Autodesk Inventor part; units mm, degrees
ref_plane "YZ Plane" through (0, 0, 0) normal (1, 0, 0) x (0, 1, 0)
ref_plane "XZ Plane" through (0, 0, 0) normal (0, 1, 0) x (-1, 0, 0)
ref_plane "XY Plane" through (0, 0, 0) normal (0, 0, 1) x (1, 0, 0)
sketch "Skizze1" plane through (0, 0, 0) normal (0, 1, 0) x (-1, 0, 0)
  line L0 (18.599, 2.8535) -> (-28.901, 2.8535)
  line L1 (-28.901, 2.8535) -> (-28.901, -12.1465)
  line L2 (-28.901, -12.1465) -> (18.599, -12.1465)
  line L3 (18.599, -12.1465) -> (18.599, 2.8535)
  line L4 (18.599, -12.1465) -> (28.599, -12.1465)
  line L5 (28.599, -12.1465) -> (28.599, 2.8535)
  line L6 (28.599, 2.8535) -> (18.599, 2.8535)
  line L7 (18.599, 2.8535) -> (18.599, -12.1465)
  point P0 (0, 0)
  dimension "d0" = 47.5
  dimension "d1" = 15
  dimension "d6" = 10
extrude "Extrusion1" add sketch "Skizze1" along normal blind 10 contours L3 L2 L1 L0
sketch "Skizze2" plane through (-18.599, 0, 2.8535) normal (0, 0, 1) x (1, 0, 0)
  line L0 (47.5, 10) -> (0, 10)
  line L1 (47.5, 0) -> (0, 10)
  line L2 (0, 10) -> (47.5, 10)
  line L3 (47.5, 10) -> (47.5, 0)
  point P0 (18.599, 0)
extrude "Extrusion2" cut sketch "Skizze2" against normal up to surface (15 mm away)
sketch "Skizze3" plane through (28.901, 0, 2.8535) normal (0.206, 0.9785, 0) x (0.9785, -0.206, 0)
  point P0 (-28.2811, 2.8535)
extrude "Extrusion3" add sketch "Skizze1" along normal blind 10 contours L6 L5 L4 L3
sketch "Skizze6" plane through (-28.599, 0, 2.8535) normal (0, 0, 1) x (1, 0, 0)
  line L0 (10, 10) -> (0, 10)
  line L1 (0, 0) -> (0, 10)
  line L2 (10, 10) -> (0, 0)
  line L3 (0, 0) -> (0, 10)
  line L4 (57.5, 0) -> (10, 10)
  line L5 (0, 10) -> (10, 10)
  point P0 (28.599, 0)
extrude "Extrusion4" cut sketch "Skizze6" against normal blind 15
sketch "Skizze7" plane through (28.901, 0, 2.8535) normal (0.206, 0.9785, 0) x (0.9785, -0.206, 0)
  line L0 (0, 15) -> (-56.2666, 15)
  line L1 (-56.2666, 0) -> (0, 0)
  line L2 (-46.5412, 15) -> (-41.5412, 15)
  line L3 (-41.5412, 15) -> (-41.5412, 0)
  line L4 (-41.5412, 0) -> (-46.5412, 0)
  line L5 (-46.5412, 0) -> (-46.5412, 15)
  line L6 (-48.5412, 15) -> (-48.5412, 0)
  line L7 (-31.5412, 15) -> (-31.5412, 0)
  line L8 (-36.5412, 15) -> (-31.5412, 15)
  line L9 (-36.5412, 0) -> (-36.5412, 15)
  line L10 (-31.5412, 0) -> (-36.5412, 0)
  line L11 (-21.5412, 15) -> (-21.5412, 0)
  line L12 (-26.5412, 15) -> (-21.5412, 15)
  line L13 (-26.5412, 0) -> (-26.5412, 15)
  line L14 (-21.5412, 0) -> (-26.5412, 0)
  line L15 (-11.5412, 15) -> (-11.5412, 0)
  line L16 (-16.5412, 15) -> (-11.5412, 15)
  line L17 (-16.5412, 0) -> (-16.5412, 15)
  line L18 (-11.5412, 0) -> (-16.5412, 0)
  point P0 (-28.2811, 2.8535)
  point P1 (-16.5412, 15)
  point P2 (-16.5412, 0)
  point P3 (-11.5412, 0)
  point P4 (-11.5412, 15)
  point P5 (-26.5412, 0)
  point P6 (-21.5412, 0)
  point P7 (-21.5412, 15)
  point P8 (-36.5412, 0)
  point P9 (-31.5412, 0)
  point P10 (-31.5412, 15)
  point P11 (-46.5412, 0)
  point P12 (-41.5412, 15)
  dimension "d11" = 5
  dimension "d12" = 2
  dimension "d15" = 10
extrude "Extrusion5" cut sketch "Skizze7" against normal blind 1.5 contours L15 L1 L17 L0 | L11 L1 L13 L0 | L7 L1 L9 L0 | L3 L1 L5 L0
properties part number "Keilvertsell"
Can you work these out from the model? Positions are in its coordinate system, mm. A direction names the side the tool comes from. Coordinates: 2 decimals unless noted, no trailing zeros. Loops run counter-clockwise (first coordinate to the right, second up) from the corner with the lowest first, then second, coordinate; pieces in that order, holes last.
Item 1: Which directions (+Z, -Z, +X, -X, +Y, -Y) give clear straight access to the entire face, cutting with the end or side of a thin tool? Please do faces 1 (the face through (12.56, 2.68, -4.54)), 2 (the face through (-11.902, 7.833, -4.751)), 3 (the face through (1, 0, -5)).
Answers below:
face 1: +Z, -Z
face 2: +Z, -Z, +Y
face 3: +Z, -Z, +X, -X, -Y
Item 2: Suppose I cut it at A-A (z = -3). Please give me the cut outline in (x, y), then the cut area to 3 significant figures.
Answers below:
outline: (-28.6, 0) - (28.9, 0) - (17.61, 2.38) - (17.3, 0.91) - (12.41, 1.94) - (12.71, 3.41) - (7.82, 4.44) - (7.51, 2.97) - (2.62, 4) - (2.93, 5.47) - (-1.96, 6.5) - (-2.27, 5.03) - (-7.17, 6.06) - (-6.86, 7.53) - (-11.75, 8.56) - (-12.06, 7.09) - (-16.95, 8.12) - (-16.64, 9.59) - (-18.6, 10) - close
area: 257 mm2
Item 3: Please list where these lines run through material, in increasing order: L1, parallel to X at y = 2.5, z = -10; L2, parallel to Y at x = -22, z = -0.5; L3, parallel to X at y = 9, z = -3.5.
Answers below:
L1: x = -26.1 to 12.52
L2: y = 0 to 6.6
L3: x = -19.6 to -16.77
Item 4: I'm going to push flat-ended pins straight in: pin 1 (3 mm diameter, centred on x = 9.5, z = -6, fed in from +Y); pin 2 (5 mm diameter, centred on y = 6, z = -5.5, fed in from -X); pin 3 (8 mm diameter, centred on x = 4.5, z = 1, fed in from -Y). Where does each tip first touch, or does it pass through?
Answers below:
pin 1: stops at y = 4.4
pin 2: stops at x = -25.1
pin 3: stops at y = 0
Item 5: Suppose I cut it at B-B (x = -6). Please give me the cut outline in (y, z).
Answers below:
outline: (0, -12.15) - (5.81, -12.15) - (5.81, 2.85) - (0, 2.85) - close
Item 6: Suppose I cut it at C-C (x = -23). Please give me the cut outline in (y, z).
Answers below:
outline: (0, -12.15) - (5.6, -12.15) - (5.6, 2.85) - (0, 2.85) - close
Item 7: If we mould it in two halves opening along Y, with no side actions, what happens to faces 4 (the face through (2.777, 4.743, -4.542)), 5 (the face through (-7, 3, 2.854)), 6 (the face through (10.302, 3.915, -4.541)), 7 (the face through (-16.794, 8.863, -4.542))? For each: released by +Y, released by -Y, zero draft, split by the parting line, or undercut.
Answers below:
face 4: undercut
face 5: zero draft
face 6: released by +Y
face 7: undercut
